Drawing for the job (mm, zero at the part's lowest x, y, z). Give positions to 0.01 mm unless a question says otherwise; leave off trailing zeros. Write each loop counter-clockwise with the first axis right and the second up, starting at its lowest first coordinate (ties: lowest second). Pieces come first, ordered by that corner, then holes. Notation, with made-up numbers: M 76,28.5 L 99,28.5 A22 cw 99,41.5 Z; hole C -11.75,56.5 d11. An arc over 180 degrees is marked long. Use CSV: the item, a comma, the result in double quotes. Start each with the question number.
1. Band-saw the part on A-A, the plane z = 11.5. List the corners of the cut face in (x, y), then the cut area to 3 significant figures.
2. Drop flat-ended pins along their axis: pin 1 Ø5 at (x, z) = (18.5, 32.5) entering from -Y; pin 2 Ø12 at (y, z) = (3, 15) entering from +X; pin 3 Ø10 at (x, z) = (3, 10) entering from +Y. Give the stop position or say it passes through.
3. Mould opens along Y. For the marked faces 1 and 2 say: pulls with the +Y half, pulls with the -Y half, needs draft (parallel to the pull), parting line crosses it, or undercut.
4. Drill centre lines: line 1 along Y through (x, z) = (10.5, 25.5); line 2 along Y through (x, z) = (13.25, 52); line 3 along X through (y, z) = (7, 36). Where is each one in solid material? Low to high. Write a range as from..to.
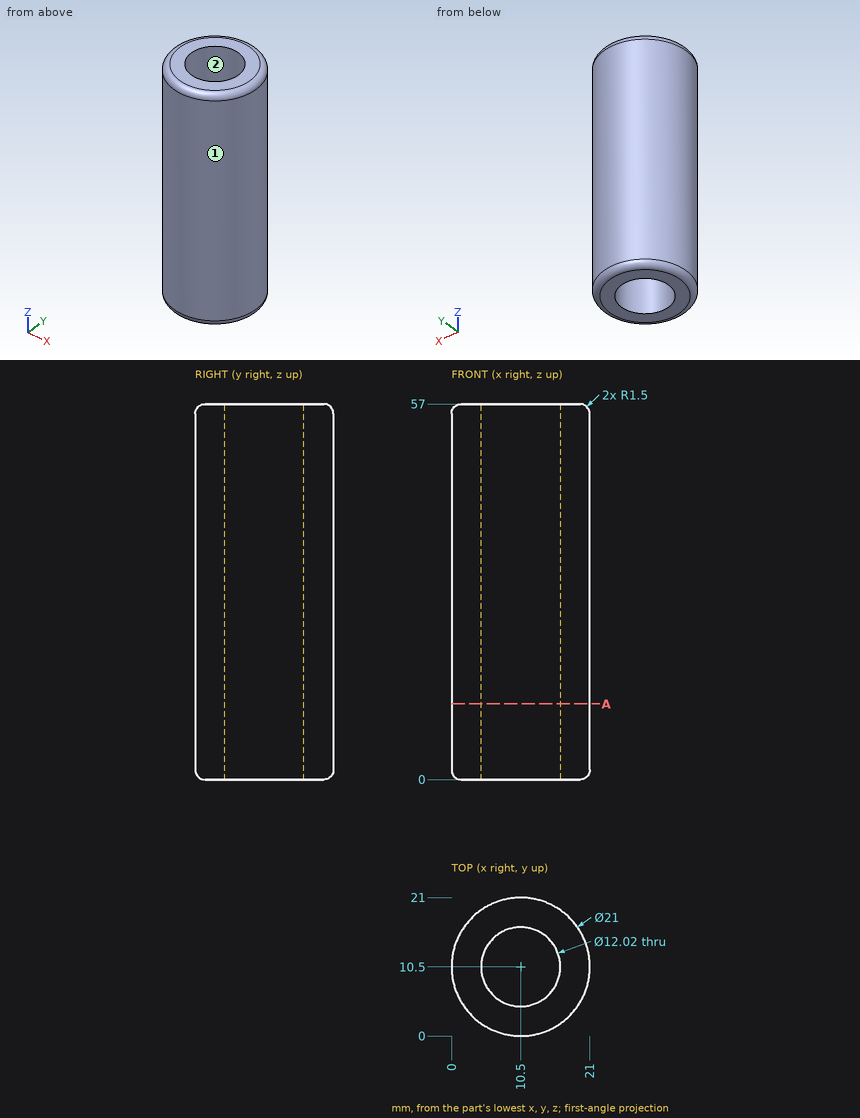
Output:
1,outline,"C 10.5,10.5 d21; hole C 10.5,10.5 d12.02"
1,area,"233 mm²"
2,pin 1,"stops at y = 1.56"
2,pin 2,"stops at x = 20.89"
2,pin 3,"stops at y = 20.7"
3,face 1,"parting line crosses it"
3,face 2,"undercut"
4,line 1,"y = 0..4.49, 16.51..21"
4,line 2,"y = 0.37..5.16, 15.84..20.63"
4,line 3,"x = 0.6..5.61, 15.39..20.4"
